from build123d import *

# Parameters (mm, degrees)
BOX_W             = 10
BOX_H             = 10
BOX_DEPTH         = 10
CYLINDER001_R     = 10
CYLINDER001_DEPTH = 5
CYLINDER002_R     = 3
CYLINDER002_DEPTH = 12
CYLINDER_R        = 20
CYLINDER_DEPTH    = 35


with BuildPart() as cube:
    # Box → Box (new body)
    with BuildSketch(Plane(origin=(2, -5, 7), x_dir=(1, 0, 0), z_dir=(0, 0, 1))):
        with Locations((5, 5)):
            Rectangle(BOX_W, BOX_H)
    extrude(amount=BOX_DEPTH)


with BuildPart() as cylinder001:
    # Cylinder001 → Cylinder001 (new body)
    with BuildSketch(Plane.XY):
        Circle(CYLINDER001_R)
    extrude(amount=CYLINDER001_DEPTH)


with BuildPart() as cylinder002:
    # Cylinder002 → Cylinder002 (new body)
    with BuildSketch(Plane.XY.offset(5)):
        Circle(CYLINDER002_R)
    extrude(amount=CYLINDER002_DEPTH)


with BuildPart() as cut:
    # Cylinder → Cylinder (new body)
    with BuildSketch(Plane.XY.offset(-35)):
        Circle(CYLINDER_R)
    extrude(amount=CYLINDER_DEPTH)

    # Fusion: union Cylinder001, Cylinder002
    add(cylinder001.part)
    add(cylinder002.part)

    # Cut: cut Cube
    add(cube.part, mode=Mode.SUBTRACT)


solid = cut.part
Geometry check sheet. Reference: the model listing, model coordinates, mm. A direction names the side the tool comes from. Give positions to 0.01 mm unless a question says otherwise; leave off trailing zeros. Loops run counter-clockwise (first coordinate to the right, second up) from the corner with the lowest first, then second, coordinate; pieces in that order, holes last. Notation, with made-up numbers: (72, 81) -> (77, 81) arc R25 cw to (77, 114) -> close; hole circle Ø4 at (85.5, 83.5). An arc over 180 degrees is marked (long way). Answer in a Markdown table with one row per item. Add a question column.
1) Cross-section at B-B on y = 0. Record the boundary of the cut face in (x, z).
2) Cross-section at C-C on z = -28. Record the boundary of the cut face in (x, y), and give its area (3 significant figures).
3) Material ranges on probe 1 along Z at (x, y) = (6, 11); probe 2 along Z at (x, y) = (6.5, -2.5); probe 3 along Y at (x, z) = (12, -12.5), recorded low to high. Write a range as from..to.
4) Set-up check for faces 1 (the face through (-4.336, -19.524, -17.745)), 2 (the face through (2, 0, 12)), 3 (the face through (-5, 9, 0)): record each of +Z, -Z, +X, -X, +Y, -Y from which the full face is reachable in a straight line by a thin tool's end or side.
5) Cross-section at A-A on x = 0. Record the boundary of the cut face in (y, z), and give its area (3 significant figures).
6) Cross-section at D-D on x = -9. Record the boundary of the cut face in (y, z), and give its area (3 significant figures).
7) Gauge pin test, flat ends, axial feed: P1, Ø1.5, axis at y = -7.5, z = -6.5, coming from the +X side; P2, Ø3.5, axis at y = -0.5, z = 13.5, coming from the +X side; P3, Ø5, axis at x = -10.5, y = -13.5, coming from the +Z side. Record the tip position at first contact, or that the pin passes through.
Outcome:
| question | item | result |
|---|---|---|
| 1 | outline | (-20, -35) -> (20, -35) -> (20, 0) -> (10, 0) -> (10, 5) -> (3, 5) -> (3, 7) -> (2, 7) -> (2, 17) -> (-3, 17) -> (-3, 5) -> (-10, 5) -> (-10, 0) -> (-20, 0) -> close |
| 2 | outline | circle Ø40 at (0, 0) |
| 2 | area | 1,260 mm^2 |
| 3 | probe 1 | z = -35..0 |
| 3 | probe 2 | z = -35..5 |
| 3 | probe 3 | y = -16..16 |
| 4 | face 1 | +Z, -Z |
| 4 | face 2 | +Z, +X, +Y, -Y |
| 4 | face 3 | +Z |
| 5 | outline | (-20, -35) -> (20, -35) -> (20, 0) -> (10, 0) -> (10, 5) -> (3, 5) -> (3, 17) -> (-3, 17) -> (-3, 5) -> (-10, 5) -> (-10, 0) -> (-20, 0) -> close |
| 5 | area | 1,570 mm^2 |
| 6 | outline | (-17.86, -35) -> (17.86, -35) -> (17.86, 0) -> (4.36, 0) -> (4.36, 5) -> (-4.36, 5) -> (-4.36, 0) -> (-17.86, 0) -> close |
| 6 | area | 1,290 mm^2 |
| 7 | P1 | stops at x = 18.83 |
| 7 | P2 | stops at x = 2 |
| 7 | P3 | stops at z = 0 |
